Verification items for the finished model (mm, model axes). A direction names the side the tool comes from. Give positions to 0.01 mm unless a question says otherwise; leave off trailing zeros. Order: outer loops, then holes, each group sorted by start corner. A loop starts at its lowest first (then second) coordinate and runs counter-clockwise, first axis right, second up.
from build123d import *

# Parameters (mm, degrees)
SKETCH041_R     = 13.97
PAD019_DEPTH    = 27.432
SKETCH042_R     = 4.445
PAD020_DEPTH    = 1.778
SKETCH043_R     = 1.524
PAD021_DEPTH    = 14.224
SKETCH044_R     = 0.8255
POCKET018_DEPTH = 5.08
SKETCH049_R     = 1.5
POCKET021_DEPTH = 5.08


with BuildPart() as part:
    # Sketch041 → Pad019 (new body)
    with BuildSketch(Plane.YZ):
        Circle(SKETCH041_R)
    extrude(amount=PAD019_DEPTH)

    # Sketch042 (on Face3 of Pad019) → Pad020 (join)
    with BuildSketch(Plane.YZ.offset(27.432)):
        Circle(SKETCH042_R)
    extrude(amount=PAD020_DEPTH)

    # Sketch043 (on Face5 of Pad020) → Pad021 (join)
    with BuildSketch(Plane.YZ.offset(29.21)):
        Circle(SKETCH043_R)
    extrude(amount=PAD021_DEPTH)

    # Sketch044 (on Face3 of Pad021) → Pocket018 (cut)
    with BuildSketch(Plane.YZ.offset(27.432)):
        with Locations((0, 5.842)):
            Circle(SKETCH044_R)
        with Locations((5.842, 0)):
            Circle(SKETCH044_R)
        with Locations((0, -5.842)):
            Circle(SKETCH044_R)
        with Locations((-5.842, 0)):
            Circle(SKETCH044_R)
    extrude(amount=-POCKET018_DEPTH, mode=Mode.SUBTRACT)

    # Sketch049 (on Face2 of Pocket018) → Pocket021 (cut)
    with BuildSketch(Plane(origin=(0, 0, 0), x_dir=(0, 1, 0), z_dir=(-1, 0, 0))):
        with Locations((0, 9.525)):
            Circle(SKETCH049_R)
        with Locations((7.9375, 0)):
            Circle(SKETCH049_R)
        with Locations((0, -9.525)):
            Circle(SKETCH049_R)
        with Locations((-7.9375, 0)):
            Circle(SKETCH049_R)
    extrude(amount=-POCKET021_DEPTH, mode=Mode.SUBTRACT)


with BuildPart() as part_1:
    # Body017 placement: moved
    add(part.part.moved(Location((-24.13, -5.33, 14.476))))


solid = part_1.part
(1) Scan lines: line 1 (X direction, y = -11, z = 27); line 2 (Z direction, x = -5, y = -5); line 3 (X direction, y = -8.75, z = 12.25). Record each from-to range of solid material in increasing order.
Solved:
line 1: x = -24.13 to 3.3
line 2: z = 0.51 to 28.44
line 3: x = -24.13 to 5.08
(2) Section check B-B, the plane x = -20. Enter the section's corners in (y, z), then the cut area to 3 significant figures.
Solved:
outline: circle Ø27.94 at (-5.33, 14.48); hole circle Ø3 at (-13.27, 14.48); hole circle Ø3 at (-5.33, 4.95); hole circle Ø3 at (-5.33, 24); hole circle Ø3 at (2.61, 14.48)
area: 585 mm2
(3) Section check D-D, the plane x = 14.5. Enter the section's corners in (y, z).
Solved:
outline: circle Ø3.05 at (-5.33, 14.48)
(4) Set-up check for faces 4 (the flat face through (-19.05, -13, 14)), 5 (the cylindrical face through (0.798, -5.985, 8.132)), 6 (the flat face through (19.304, -5, 14)): record each of +Z, -Z, +X, -X, +Y, -Y from which the full face is reachable in a straight line by a thin tool's end or side.
Solved:
face 4: -X
face 5: +X
face 6: +Z, -Z, +X, +Y, -Y
(5) Section check C-C, the plane z = 17. Enter the section's corners in (x, y), then the cut area to 3 significant figures.
Solved:
outline: (-24.13, -19.07) - (3.3, -19.07) - (3.3, -8.99) - (5.08, -8.99) - (5.08, -1.67) - (3.3, -1.67) - (3.3, 8.41) - (-24.13, 8.41) - close
area: 767 mm2
(6) Section check A-A, the plane y = -5.33. Enter the section's corners in (x, z), then the cut area to 3 significant figures.
Solved:
outline: (-24.13, 0.51) - (3.3, 0.51) - (3.3, 7.81) - (-1.78, 7.81) - (-1.78, 9.46) - (3.3, 9.46) - (3.3, 10.03) - (5.08, 10.03) - (5.08, 12.95) - (19.3, 12.95) - (19.3, 16) - (5.08, 16) - (5.08, 18.92) - (3.3, 18.92) - (3.3, 19.49) - (-1.78, 19.49) - (-1.78, 21.14) - (3.3, 21.14) - (3.3, 28.45) - (-24.13, 28.45) - (-24.13, 25.5) - (-19.05, 25.5) - (-19.05, 22.5) - (-24.13, 22.5) - (-24.13, 6.45) - (-19.05, 6.45) - (-19.05, 3.45) - (-24.13, 3.45) - close
area: 778 mm2
(7) Release check for a two-part mould opening along Z. For faces 1 (the cylindrical face through (0.798, 0.405, 15.294)), 2 (the cylindrical face through (4.179, -6.294, 10.137)), 3 (the flat face through (5.08, -3, 15)) record: pulls with the +Z half, pulls with the -Z half, needs draft (parallel to the pull), parting line crosses it, or undercut.
Solved:
face 1: undercut
face 2: parting line crosses it
face 3: needs draft
(8) Go/stop test with flat-tipped pins: pin 1 (5 mm diameter, centred on x = -10, z = 23, fed in from +Y); pin 2 (5 mm diameter, centred on y = -13.27, z = 14.48, fed in from +X); pin 3 (0.9 mm diameter, centred on y = -6, z = 24.5, fed in from -X). Record where each tip stops, or that it passes through.
Solved:
pin 1: stops at y = 7.27
pin 2: stops at x = 3.3
pin 3: stops at x = -19.05
